Can you work these out from the model? Positions are in its coordinate system, mm. Face numbers are marked on the shaded views. A direction names the side the tool comes from. Coordinates: 2 decimals unless noted, no trailing zeros. Order: outer loops, then holes, each group sorted by start corner. A loop starts at its lowest first (then second) coordinate and runs counter-clockwise, first axis right, second up. Notation, with made-up numbers: (34.5, -1.5) -> (45.5, -1.5) arc R13 ccw to (45.5, 23.5) -> close; hole circle Ø7 at (31, -10). An arc over 180 degrees is marked (long way). Return JSON: item names as keys, results as strings. Group by question number.
1) If we section it at D-D, the plane y = 34: Please give me the cut outline in (x, z).
2) If we section it at A-A, the plane z = 109: Please give me the cut outline in (x, y), then the cut area to 3 significant figures.
3) For pin 1 (10 mm diameter, centred on x = -1.5, y = -14, fed in from +Z); pin 2 (5 mm diameter, centred on y = 6.5, z = 93, fed in from -X); pin 3 (4 mm diameter, centred on x = -9.5, y = 61, fed in from +Z); pin 4 (8 mm diameter, centred on x = 23.75, y = 0, fed in from -Z), each with a flat end and sliding along its axis, tell me the tip position at first contact or that it passes through.
4) If we section it at C-C, the plane x = 0: State how many separate pieces and enclosed holes the cut face has, then the cut area to 3 significant figures.
5) If we section it at B-B, the plane y = -23.75: Please give me the cut outline in (x, z).
6) If I drill on probe 1 along Z at (x, y) = (-20, 59.9); probe 2 along X at (y, z) = (62.15, 114.75), over which ranges is the centre line in solid material (lowest first)? Write a range as from..to.
7) For the marked faces 4, 5, 6 and 7, which set-ups out of +Z, -Z, +X, -X, +Y, -Y let a thin tool reach every point of the face, with its end or its side?
8) Thinking about a two-plate mould opening in Y: for the marked faces 1, 2 and 3, which applies, +Y half, -Y half, draft (parallel to the pull), parting line (faces both ways), or undercut?
from build123d import *

# Parameters (mm, degrees)
SKETCH1_R                 = 12.5
SKETCH1_R_2               = 10
SKETCH9_W                 = 50
SKETCH9_H                 = 50
SKETCH9_R                 = 10
BOSS_EXTRUDE5_DEPTH       = 5
FILLET1_R                 = 5
HOLE1_D                   = 5
BOSS_EXTRUDE7_START       = -5
SKETCH15_R                = 28.75
SKETCH15_R_2              = 10
BOSS_EXTRUDE7_DEPTH       = 5
HOLE2_D                   = 5
HOLE2_DEPTH               = 5
CIRPATTERN2_COUNT         = 4
BOSS_EXTRUDE8_REACH       = 135.487
BOSS_EXTRUDE8_END_RADIUS  = 12.5
SKETCH20_R                = 10
BOSS_EXTRUDE9_DEPTH       = 4
HOLE3_D                   = 5
HOLE3_DEPTH               = 5
HOLE5_D                   = 15
HOLE5_DEPTH               = 22.75
BOSS_EXTRUDE10_REACH      = 145.888
BOSS_EXTRUDE10_END_RADIUS = 12.5
SKETCH32_R                = 10
HOLE6_REACH               = 145.888
HOLE6_BORE_R              = 7.5


with BuildPart() as part:
    # Sweep1: sweep along a path in Sketch3
    with BuildLine(Plane(origin=(0, 0, 0), x_dir=(0, 0, -1), z_dir=(1, 0, 0))) as sweep1_path:
        Line((0, 0), (-76, 0))
        ThreePointArc((-76, 0), (-89.258252147, 5.491747853), (-94.75, 18.75))
        Line((-94.75, 18.75), (-94.75, 63.75))
    # Sketch1 → Sweep1 (sweep)
    with BuildSketch(Plane.XY):
        Circle(SKETCH1_R)
        Circle(SKETCH1_R_2, mode=Mode.SUBTRACT)
    sweep(path=sweep1_path.line)

    # Sketch9 → Boss-Extrude5 (add)
    with BuildSketch(Plane(origin=(0, 63.75, 0), x_dir=(1, 0, 0), z_dir=(0, 1, 0))):
        with Locations((0, -94.75)):
            Rectangle(SKETCH9_W, SKETCH9_H)
        with Locations(Location((0, -94.75, 0), (0, 0, 270))):
            Circle(SKETCH9_R, mode=Mode.SUBTRACT)
    extrude(amount=-BOSS_EXTRUDE5_DEPTH)

    # Fillet1
    fillet1_edges = [part.edges().sort_by_distance(p)[0] for p in [
        (25, 61.25, 69.75),
        (25, 61.25, 119.75),
        (-25, 61.25, 119.75),
        (-25, 61.25, 69.75),
    ]]
    fillet(fillet1_edges, radius=FILLET1_R)

    # Hole1 (through all)
    with Locations(Plane(origin=(0, 63.75, 0), x_dir=(1, 0, 0), z_dir=(0, 1, 0))):
        with Locations((-20, -74.75), (20, -74.75), (20, -114.75), (-20, -114.75)):
            Hole(HOLE1_D / 2)

    # Sketch15 → Boss-Extrude7 (add)
    with BuildSketch(Plane(origin=(0, 0, 0), x_dir=(-1, 0, 0), z_dir=(0, 0, -1)).offset(BOSS_EXTRUDE7_START)):
        Circle(SKETCH15_R)
        with Locations(Location((0, 0, 0), (0, 0, 180))):
            Circle(SKETCH15_R_2, mode=Mode.SUBTRACT)
    extrude(amount=BOSS_EXTRUDE7_DEPTH)

    # Hole2
    with Locations(Plane(origin=(0, 0, 0), x_dir=(-1, 0, 0), z_dir=(0, 0, -1))):
        with Locations((23.75, 0)):
            hole2 = Hole(HOLE2_D / 2, depth=HOLE2_DEPTH)

    # CirPattern2: Hole2 ×4 about axis
    cirpattern2_axis = Axis((0, 0, 0), (0, 0, 1))
    for i in range(1, CIRPATTERN2_COUNT):
        add(hole2.rotate(cirpattern2_axis, i * 360 / CIRPATTERN2_COUNT), mode=Mode.SUBTRACT)

    # Boss-Extrude8: up to this cylinder (the profile starts outside it)
    boss_extrude8_end = Plane(origin=(0, 0, 42.75), z_dir=(0, 0, 1)) * Cylinder(BOSS_EXTRUDE8_END_RADIUS, 296.974, mode=Mode.PRIVATE)
    # Sketch20 → Boss-Extrude8 (add, up to the surface)
    with BuildSketch(Plane(origin=(0, 22.75, 0), x_dir=(1, 0, 0), z_dir=(0, 1, 0)), mode=Mode.PRIVATE) as boss_extrude8_sk1:
        with Locations(Location((0, -42.75, 0), (0, 0, 270))):
            Circle(SKETCH20_R)
    boss_extrude8_tool1 = extrude(boss_extrude8_sk1.sketch, amount=-BOSS_EXTRUDE8_REACH, mode=Mode.PRIVATE) - boss_extrude8_end
    add(boss_extrude8_tool1.solids().sort_by_distance((0, 22.75, 42.75))[0])

    # Sketch21 → Boss-Extrude9 (add)
    with BuildSketch(Plane(origin=(0, 22.75, 0), x_dir=(1, 0, 0), z_dir=(0, 1, 0))):
        with BuildLine():
            Line((5.357142857, -31.456151214), (19.642857143, -38.232460485))
            ThreePointArc((19.642857143, -38.232460485), (22.5, -42.75), (19.642857143, -47.267539515))
            Line((19.642857143, -47.267539515), (5.357142857, -54.043848786))
            ThreePointArc((5.357142857, -54.043848786), (0, -55.25), (-5.357142857, -54.043848786))
            Line((-5.357142857, -54.043848786), (-19.642857143, -47.267539515))
            ThreePointArc((-19.642857143, -47.267539515), (-22.5, -42.75), (-19.642857143, -38.232460485))
            Line((-19.642857143, -38.232460485), (-5.357142857, -31.456151214))
            ThreePointArc((-5.357142857, -31.456151214), (0, -30.25), (5.357142857, -31.456151214))
        make_face()
    extrude(amount=-BOSS_EXTRUDE9_DEPTH)

    # Hole3
    with Locations(Plane(origin=(0, 22.75, 0), x_dir=(1, 0, 0), z_dir=(0, 1, 0))):
        with Locations((-17.5, -42.75), (17.5, -42.75)):
            Hole(HOLE3_D / 2, depth=HOLE3_DEPTH)

    # Hole5
    with Locations(Plane(origin=(0, 22.75, 0), x_dir=(1, 0, 0), z_dir=(0, 1, 0))):
        with Locations((0, -42.75)):
            Hole(HOLE5_D / 2, depth=HOLE5_DEPTH)

    # Boss-Extrude10: up to this cylinder (the profile starts outside it)
    boss_extrude10_end = Plane(origin=(0, 46.25, 94.75), z_dir=(0, 1, 0)) * Cylinder(BOSS_EXTRUDE10_END_RADIUS, 317.776, mode=Mode.PRIVATE)
    # Sketch32 → Boss-Extrude10 (add, up to the surface)
    with BuildSketch(Plane.XY.offset(125.75), mode=Mode.PRIVATE) as boss_extrude10_sk1:
        with Locations((0, 46.25)):
            Circle(SKETCH32_R)
    boss_extrude10_tool1 = extrude(boss_extrude10_sk1.sketch, amount=-BOSS_EXTRUDE10_REACH, mode=Mode.PRIVATE) - boss_extrude10_end
    add(boss_extrude10_tool1.solids().sort_by_distance((0, 46.25, 125.75))[0])

    # Hole6 bore → Hole6 (cut, up to next)
    with BuildSketch(Plane.XY.offset(125.75), mode=Mode.PRIVATE) as hole6_sk1:
        with Locations((0, 46.25)):
            Circle(HOLE6_BORE_R)
    hole6_tool1 = extrude(hole6_sk1.sketch, amount=-HOLE6_REACH, mode=Mode.PRIVATE) & part.part
    add(hole6_tool1.solids().sort_by_distance((0, 46.25, 125.75))[0], mode=Mode.SUBTRACT)


solid = part.part
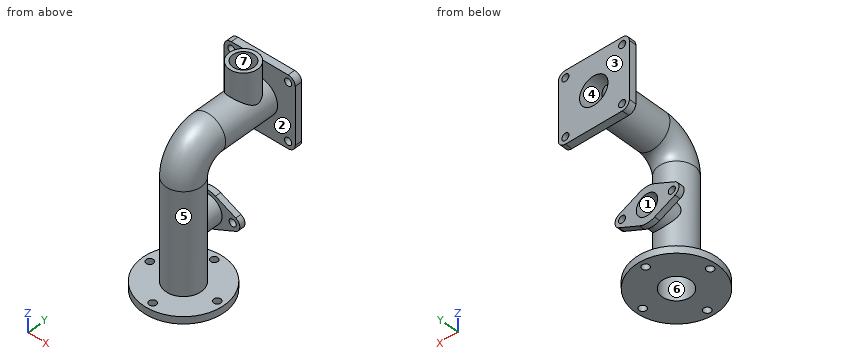
Result sheet:
{
 "1": {"outline": "circle Ø25 at (0, 94.75); hole circle Ø20 at (0, 94.75)"},
 "2": {"outline": "(-25, 58.75) -> (25, 58.75) -> (25, 63.75) -> (-25, 63.75) -> close; circle Ø20 at (0, 46.25); hole circle Ø15 at (0, 46.25)", "area": "387 mm2"},
 "3": {"pin 1": "stops at z = 90.23", "pin 2": "stops at x = -12.5", "pin 3": "stops at z = 119.75", "pin 4": "stops at z = 0"},
 "4": {"separate pieces": "6", "enclosed holes": "0", "area": "1,080 mm2"},
 "5": {"outline": "(-16.2, 0) -> (-2.5, 0) -> (-2.5, 5) -> (-16.2, 5) -> close; (2.5, 0) -> (16.2, 0) -> (16.2, 5) -> (2.5, 5) -> close"},
 "6": {"probe 1": "z = 69.75..72.25, 77.25..112.25, 117.25..119.75", "probe 2": "x = -25..-22.5, -17.5..17.5, 22.5..25"},
 "7": {"face 4": "+Y", "face 5": "none", "face 6": "-Z", "face 7": "+Z"},
 "8": {"face 1": "draft", "face 2": "undercut", "face 3": "+Y half"}
}
